Verification items for this drawing (mm, ordinates from the low corner). A direction names the side the tool comes from. Coordinates: 2 decimals unless noted, no trailing zeros. Write each loop counter-clockwise with the first axis right and the second up, starting at its lowest first coordinate (ties: lowest second). Pieces come first, ordered by that corner, then holes. Notation, with made-up numbers: M 75,21.25 L 112,21.25 A11 ccw 112,29.25 Z; hole C -17,2 d7. An arc over 180 degrees is marked long. Answer as CSV lines item,"result". Start each with the question number.
1) Go/stop test with flat-tipped pins: pin 1 Ø9.5 at (y, z) = (12.7, 35.72) entering from +X (1 decimal); pin 2 Ø11.5 at (x, z) = (31, 13.5) entering from +Y (1 decimal). Record where each tip stops, or that it passes through.
2) Section check B-B (z = 13.5). State how many separate pieces and enclosed holes the cut face has.
3) Material ranges on L1, parallel to Z at x = 12.7, y = 2.15 (1 decimal); L2, parallel to Y at x = 34.5, z = 36 (1 decimal), recorded low to high. Write a range as [from, to].
4) Access from +Z, -Z, +X, -X, +Y, -Y to the whole of each face (thin tool, end or side, straight path). Record for the marked faces 1 and 2.
5) Section check A-A (x = 38.1). Record the cut outline in (y, z) (1 decimal).
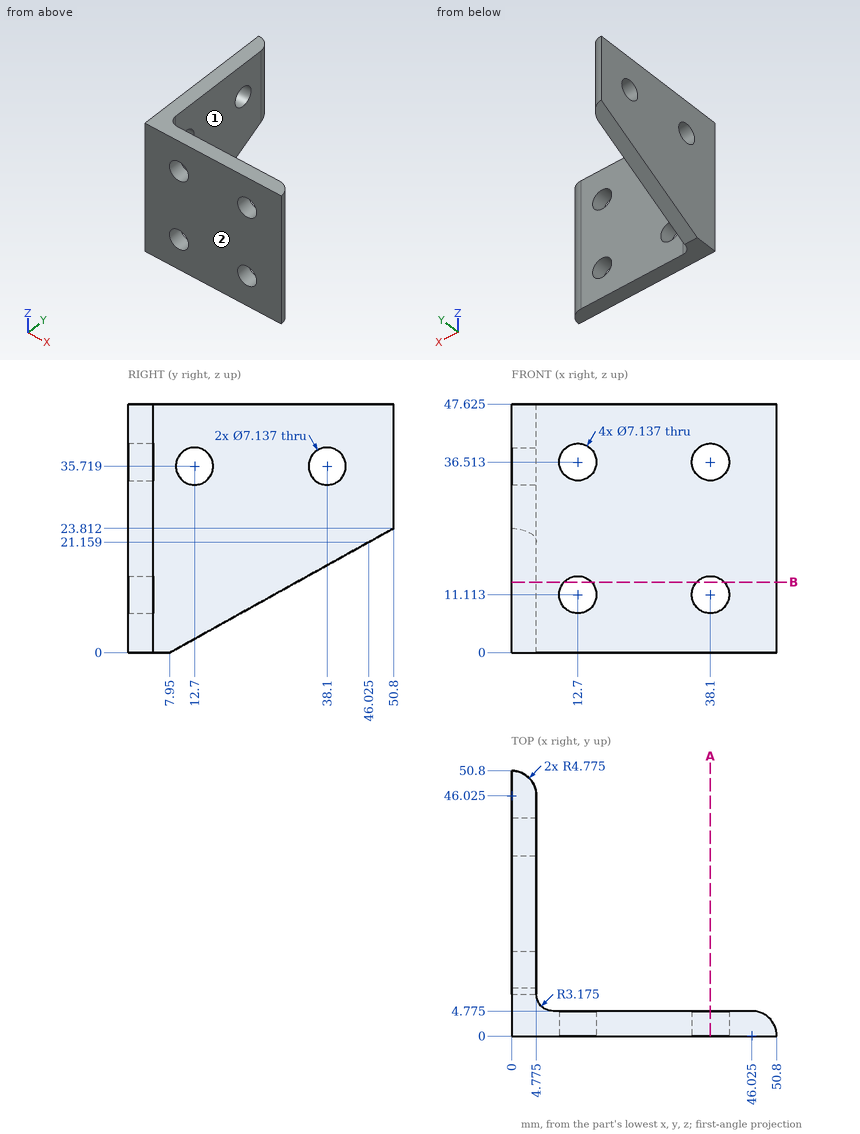
Results found:
1,pin 1,"stops at x = 4.8"
1,pin 2,"stops at y = 4.8"
2,separate pieces,"3"
2,enclosed holes,"0"
3,L1,"z = [0, 7.5], [14.7, 32.9], [40.1, 47.6]"
3,L2,"y = [0, 4.8]"
4,face 1,"+Z, -Z, +X, +Y"
4,face 2,"+Z, -Z, +X, -X, -Y"
5,outline,"M 0,0 L 4.8,0 L 4.8,7.5 L 0,7.5 Z; M 0,14.7 L 4.8,14.7 L 4.8,32.9 L 0,32.9 Z; M 0,40.1 L 4.8,40.1 L 4.8,47.6 L 0,47.6 Z"
